Work out the finished part from the listing and answer in its coordinate system (mm). Face numbers are marked on the shaded views. A direction names the side the tool comes from. Coordinates: 2 decimals unless noted, no trailing zeros. Order: outer loops, then holes, each group sorted by start corner. A loop starts at its lowest first (then second) coordinate and runs counter-clockwise, first axis right, second up. Notation, with made-up numbers: M 51,-2 L 109,-2 A23 cw 109,10 Z; hole C 12.25,35.25 d3. An arc over 180 degrees is marked long. Use a Markdown table: item, result.
Autodesk Inventor part; units mm, degrees
ref_plane "YZ Plane" through (0, 0, 0) normal (1, 0, 0) x (0, 1, 0)
ref_plane "XZ Plane" through (0, 0, 0) normal (0, 1, 0) x (-1, 0, 0)
ref_plane "XY Plane" through (0, 0, 0) normal (0, 0, 1) x (1, 0, 0)
sketch "Sketch1" plane through (0, 0, 0) normal (0, 1, 0) x (-1, 0, 0)
  circle A0 centre (0, 19.5421) radius 4.775
  circle A1 centre (-37.22, 0) radius 4.775
  circle A2 centre (38.1926, 0) radius 4.775
  circle A3 centre (38.1926, 19.5421) radius 4.775
  circle A4 centre (-37.22, 19.5421) radius 4.775
  line L0 (52.9676, 0) -> (52.9676, -4.775)
  line L1 (52.9676, -9.775) -> (-51.995, -9.775)
  line L2 (-51.995, -9.775) -> (-51.995, 24.3171)
  line L3 (-51.995, 24.3171) -> (-51.995, 29.3171)
  line L4 (-51.995, 29.3171) -> (52.9676, 29.3171)
  line L5 (52.9676, 29.3171) -> (52.9676, -9.775)
  line L6 (-8.8, 0) -> (8.8, 0)
  line L7 (8.8, 0) -> (8.8, 3.95)
  line L8 (8.8, 3.95) -> (-8.8, 3.95)
  line L9 (-8.8, 3.95) -> (-8.8, 0)
  point P0 (0, 0)
  point P1 (0, 0)
  dimension "d6" = 9.55
  dimension "d8" = 9.55
  dimension "d10" = 9.55
  dimension "d11" = 9.55
  dimension "d12" = 9.55
  dimension "d24" = 5
  dimension "d26" = 17.6
  dimension "d27" = 3.95
extrude "Extrusion1" add sketch "Sketch1" along normal blind 7
extrude "Extrusion2" add sketch "Sketch1" along normal blind 80 contours A2 | A3
extrude "Extrusion3" add sketch "Sketch1" along normal blind 80 contours A1
extrude "Extrusion4" add sketch "Sketch1" along normal blind 80 contours A4
extrude "Extrusion5" add sketch "Sketch1" along normal blind 80 contours A0
fillet "Fillet1" radius 2 3 edges at (51.995, 7, 9.771) (-0.4863, 7, -9.775) (-0.4863, 7, 29.3171)
fillet "Fillet2" radius 2 3 edges at (-0.4863, 0, 29.3171) (-0.4863, 0, -9.775) (51.995, 0, 9.771)
properties part number "BluetoothBase"
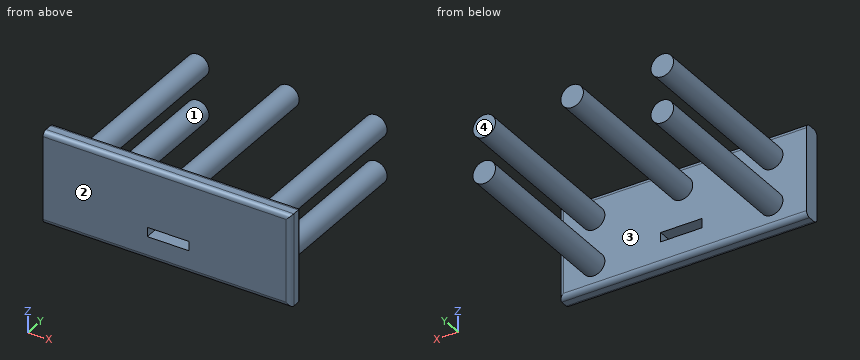
(1) A cutting plane is placed at A-A (x = 37.22). Determine the outline of the cut face in (y, z) (3 decimals).
Conclusion:
| item | result |
|---|---|
| outline | M 0,-7.775 A2 ccw 2,-9.775 L 5,-9.775 A2 ccw 7,-7.775 L 7,-4.775 L 80,-4.775 L 80,4.775 L 7,4.775 L 7,14.767 L 80,14.767 L 80,24.317 L 7,24.317 L 7,27.317 A2 ccw 5,29.317 L 2,29.317 A2 ccw 0,27.317 Z |
(2) Given P1, Ø4, axis at x = -8.5, z = -2.5, coming from the +Y side; P2, Ø4, axis at y = 49.5, z = 13.5, coming from the +X side; P3, Ø12, axis at x = 30, y = 26, coming from the +Z side, each flat-ended and moving along its own axis, determine where each tip first touches the part or whether it passes through.
Conclusion:
| item | result |
|---|---|
| P1 | y = 7 |
| P2 | x = 39.76 |
| P3 | z = 24.16 |
(3) A cutting plane is placed at C-C (y = 30). Determine the outline of the cut face in (x, z) (3 decimals).
Conclusion:
| item | result |
|---|---|
| outline | C -38.193,0 d9.55; C -38.193,19.542 d9.55; C 0,19.542 d9.55; C 37.22,0 d9.55; C 37.22,19.542 d9.55 |
(4) Straight lines are drawn through the part: L1, parallel to X at y = 30, z = 18.5; L2, parallel to X at y = 64, z = 21; L3, parallel to Y at x = 14, z = 15. For each, find the intervals that lie inside material, in ascending order.
Conclusion:
| item | result |
|---|---|
| L1 | -42.85 to -33.53, -4.66 to 4.66, 32.56 to 41.88 |
| L2 | -42.74 to -33.65, -4.55 to 4.55, 32.67 to 41.77 |
| L3 | 0 to 7 |
(5) Which of the six approach directions +Z, -Z, +X, -X, +Y, -Y give full straight-line access (tool end or side, diameter ignored) to the marked faces 3 and 4?
Conclusion:
| item | result |
|---|---|
| face 3 | +Y |
| face 4 | +Z, -Z, +X, -X, +Y |
(6) A cutting plane is placed at D-D (x = -19). Determine the outline of the cut face in (y, z) (3 decimals), then the cut area to 3 significant figures.
Conclusion:
| item | result |
|---|---|
| outline | M 0,-7.775 A2 ccw 2,-9.775 L 5,-9.775 A2 ccw 7,-7.775 L 7,27.317 A2 ccw 5,29.317 L 2,29.317 A2 ccw 0,27.317 Z |
| area | 270 mm2 |
(7) A cutting plane is placed at B-B (z = 8). Determine the outline of the cut face in (x, y) (3 decimals), then the cut area to 3 significant figures.
Conclusion:
| item | result |
|---|---|
| outline | M -52.968,0 L 49.995,0 A2 ccw 51.995,2 L 51.995,5 A2 ccw 49.995,7 L -52.968,7 Z |
| area | 733 mm2 |
(8) Determine the mould class of the marked faces 1 and 2 for opening direction X: pulls with the +X half, pulls with the -X half, needs draft (parallel to the pull), parting line crosses it, or undercut.
Conclusion:
| item | result |
|---|---|
| face 1 | undercut |
| face 2 | needs draft |
